from build123d import *

# Parameters (mm, degrees)
SKETCH1_R           = 15
BOSS_EXTRUDE1_DEPTH = 200
SKETCH2_R           = 25
BOSS_EXTRUDE2_DEPTH = 25
SKETCH3_R           = 75
BOSS_EXTRUDE3_DEPTH = 10
SKETCH4_R           = 7.5
CUT_EXTRUDE1_DEPTH  = 1


with BuildPart() as part:
    # Sketch1 → Boss-Extrude1 (new body)
    with BuildSketch(Plane.XY):
        Circle(SKETCH1_R)
    extrude(amount=BOSS_EXTRUDE1_DEPTH)

    # Sketch2 → Boss-Extrude2 (add)
    with BuildSketch(Plane.XY.offset(200)):
        Circle(SKETCH2_R)
    extrude(amount=BOSS_EXTRUDE2_DEPTH)

    # Sketch3 → Boss-Extrude3 (add)
    with BuildSketch(Plane(origin=(0, 0, 0), x_dir=(-1, 0, 0), z_dir=(0, 0, -1))):
        Circle(SKETCH3_R)
    extrude(amount=BOSS_EXTRUDE3_DEPTH)

    # Sketch4 → Cut-Extrude1 (cut)
    with BuildSketch(Plane(origin=(0, 0, -10), x_dir=(-1, 0, 0), z_dir=(0, 0, -1))):
        with Locations((0, 30)):
            Circle(SKETCH4_R)
        with Locations((0, -30)):
            Circle(SKETCH4_R)
    extrude(amount=-CUT_EXTRUDE1_DEPTH, mode=Mode.SUBTRACT)


solid = part.part
The listing builds one solid part. Answer for the finished solid, in the listing's coordinates (mm). A direction names the side the tool comes from. Round coordinates to 2 decimals unless told otherwise and drop trailing zeros. Order: outer loops, then holes, each group sorted by start corner. A loop starts at its lowest first (then second) coordinate and runs counter-clockwise, first axis right, second up. Notation, with made-up numbers: (89, 46) -> (131, 46) arc R19 cw to (131, 59) -> close; hole circle Ø3 at (29.5, 79). An arc over 180 degrees is marked (long way). Put each result on its own line as item: value.
Q1. Section C-C, the plane z = 17 is taken. Write down the section's boundary in (x, y), and give its area (3 significant figures).
Results list:
outline: circle Ø30 at (0, 0)
area: 707 mm^2
Q2. Section B-B, the plane x = 0 is taken. Write down the section's boundary in (y, z), and give its area (3 significant figures).
Results list:
outline: (-75, -10) -> (-37.5, -10) -> (-37.5, -9) -> (-22.5, -9) -> (-22.5, -10) -> (22.5, -10) -> (22.5, -9) -> (37.5, -9) -> (37.5, -10) -> (75, -10) -> (75, 0) -> (15, 0) -> (15, 200) -> (25, 200) -> (25, 225) -> (-25, 225) -> (-25, 200) -> (-15, 200) -> (-15, 0) -> (-75, 0) -> close
area: 8,720 mm^2
Q3. Section D-D, the plane y = 30 is taken. Write down the section's boundary in (x, z), and give its area (3 significant figures).
Results list:
outline: (-68.74, -10) -> (-7.5, -10) -> (-7.5, -9) -> (7.5, -9) -> (7.5, -10) -> (68.74, -10) -> (68.74, 0) -> (-68.74, 0) -> close
area: 1,360 mm^2
Q4. Determine the mould class of faces 1 (the cylindrical face through (9.764, 74.362, -4.93)), 2 (the cylindrical face through (1.63, 22.68, -9.51)), 3 (the flat face through (1, 1, -10)) for opening direction Y: pulls with the +Y half, pulls with the -Y half, needs draft (parallel to the pull), parting line crosses it, or undercut.
Results list:
face 1: parting line crosses it
face 2: undercut
face 3: needs draft
Q5. Consider line 1 along Y through (x, z) = (0, -9.7); line 2 along Z through (x, y) = (-20.5, 11); line 3 along Z through (x, y) = (27.5, -38). Determine where each line is inside the solid, lowest interval first.
Results list:
line 1: -75 to -37.5, -22.5 to 22.5, 37.5 to 75
line 2: -10 to 0, 200 to 225
line 3: -10 to 0
Q6. Each of these flat-tipped pins is pushed along its axis until it touches: P1, Ø10, axis at x = 10.5, y = 37, coming from the +Z side; P2, Ø16.5, axis at x = 1, y = -26.5, coming from the -Z side; P3, Ø12, axis at x = 0, y = -30, coming from the -Z side; P4, Ø2, axis at y = -17, z = 186.5, coming from the -X side (1 decimal). Where does it stop, or does it pass through?
Results list:
P1: z = 0
P2: z = -10
P3: z = -9
P4: through
Q7. Which of the six approach directions +Z, -Z, +X, -X, +Y, -Y give full straight-line access (tool end or side, diameter ignored) to faces 4 (the cylindrical face through (1.63, -37.32, -9.51)), 5 (the flat face through (11, -11, 200)), 6 (the cylindrical face through (23.846, 7.509, 212.325))?
Results list:
face 4: -Z
face 5: none
face 6: +Z
Q8. Section A-A, the plane y = 0 is taken. Write down the section's boundary in (x, z).
Results list:
outline: (-75, -10) -> (75, -10) -> (75, 0) -> (15, 0) -> (15, 200) -> (25, 200) -> (25, 225) -> (-25, 225) -> (-25, 200) -> (-15, 200) -> (-15, 0) -> (-75, 0) -> close
